```python
from build123d import *

# Parameters (mm, degrees)
F0_W     = 76.2
F0_H     = 76.2
F1_DEPTH = 50.8
F2_R     = 25.4
F3_R     = 25.4
F4_DEPTH = 45.72


with BuildPart() as f1:
    # F0 (on Top) → F1 (new body)
    with BuildSketch(Plane.XY):
        Rectangle(F0_W, F0_H)
    extrude(amount=F1_DEPTH)

    # F2
    f2_edges = [f1.edges().sort_by_distance(p)[0] for p in [
        (-38.1, -38.1, 25.4),
        (38.1, -38.1, 25.4),
        (-38.1, 38.1, 25.4),
        (38.1, 38.1, 25.4),
    ]]
    fillet(f2_edges, radius=F2_R)

    # F3 (on face) → F4 (cut)
    with BuildSketch(Plane.XY.offset(50.8)):
        Circle(F3_R)
    extrude(amount=-F4_DEPTH, mode=Mode.SUBTRACT)


solid = f1.part
```
CAD build for the part. Positions are in the model's coordinates, mm. A direction names the side the tool comes from. Give positions to 0.01 mm unless a question says otherwise; leave off trailing zeros. Order: outer loops, then holes, each group sorted by start corner. A loop starts at its lowest first (then second) coordinate and runs counter-clockwise, first axis right, second up. Notation, with made-up numbers: M 56,-34 L 82,-34 A13 ccw 82,-27 Z; hole C 52,23.5 d7. An arc over 180 degrees is marked long. Put each result on its own line as item: value. Start each with the question number.
(1) Which spindle directions (+Z, -Z, +X, -X, +Y, -Y) get a long thin tool onto all of the face, cutting with end or side? Do faces 4 (the flat face through (-1, 1, 0)), 5 (the flat face through (0, 0, 5.08)). Say none if no direction does.
(2) Saw through at A-A, the plane y = 0. Write the cut outline in (x, z).
(3) Saw through at D-D, the plane x = -32. Write the cut outline in (y, z), then the cut area to 3 significant figures.
(4) Mould opens along X. For faces 1 (the cylindrical face through (-5.506, -24.796, 28.26)), 2 (the flat face through (38.1, 0, 25)), 3 (the flat face through (-38.1, 0, 25)) say: +X half, -X half, draft (parallel to the pull), parting line (faces both ways), or undercut.
(5) Saw through at B-B, the plane z = 28. Write the cut outline in (x, y), then the cut area to 3 significant figures.
(6) Flat gauge pins, fed straight in: pin 1 Ø5 at (x, z) = (29, 12.5) entering from +Y; pin 2 Ø5 at (y, z) = (18.5, 30.5) entering from -X. Where does each tip first touch, or does it go through?
(7) Drill centre lines: line 1 along Y through (x, z) = (0, 27); line 2 along X through (y, z) = (-22.5, 47.5); line 3 along X through (y, z) = (3, 31.5). Where is each one in solid material? Low to high.
Check result:
1. face 4: -Z, +X, -X, +Y, -Y
1. face 5: +Z
2. outline: M -38.1,0 L 38.1,0 L 38.1,50.8 L 25.4,50.8 L 25.4,5.08 L -25.4,5.08 L -25.4,50.8 L -38.1,50.8 Z
3. outline: M -29.21,0 L 29.21,0 L 29.21,50.8 L -29.21,50.8 Z
3. area: 2,970 mm2
4. face 1: undercut
4. face 2: +X half
4. face 3: -X half
5. outline: M -38.1,-12.7 A25.4 ccw -12.7,-38.1 L 12.7,-38.1 A25.4 ccw 38.1,-12.7 L 38.1,12.7 A25.4 ccw 12.7,38.1 L -12.7,38.1 A25.4 ccw -38.1,12.7 Z; hole C 0,0 d50.8
5. area: 3,230 mm2
6. pin 1: stops at y = 34.02
6. pin 2: stops at x = -37.88
7. line 1: y = -38.1 to -25.4, 25.4 to 38.1
7. line 2: x = -36.13 to -11.79, 11.79 to 36.13
7. line 3: x = -38.1 to -25.22, 25.22 to 38.1
